Work out the finished part from the listing and answer in its coordinate system (mm). Face numbers are marked on the shaded views. A direction names the side the tool comes from. Coordinates: 2 decimals unless noted, no trailing zeros. Write each loop counter-clockwise with the first axis right and the second up, starting at its lowest first coordinate (ties: lowest second). Pieces come first, ordered by that corner, then holes. Notation, with made-up numbers: (-22.75, 8.5) - (12.25, 8.5) arc R18 cw to (12.25, 33.5) - close; hole circle Ø3 at (30, 51.5). An arc over 180 degrees is marked (long way). One line per item, written item: value.
```python
from build123d import *

# Parameters (mm, degrees)
ESQUISSE1_W             = 28
ESQUISSE1_H             = 23
BOSS_EXTRU_1_DEPTH      = 2
ESQUISSE2_R             = 2
ENL_V_MAT_EXTRU_1_DEPTH = 37.290494623
CHANFREIN1_SIZE         = 1


with BuildPart() as part:
    # Esquisse1 → Boss.-Extru.1 (new body)
    with BuildSketch(Plane.XY):
        with Locations((14, 11.5)):
            Rectangle(ESQUISSE1_W, ESQUISSE1_H)
    extrude(amount=BOSS_EXTRU_1_DEPTH)

    # Esquisse2 → Enlèv. mat.-Extru.1 (cut, through all)
    with BuildSketch(Plane.XY.offset(2)):
        with Locations((6, 4)):
            Circle(ESQUISSE2_R)
        with Locations(Location((22, 4, 0), (0, 0, 180))):
            Circle(ESQUISSE2_R)
        with BuildLine():
            Line((8.2, 19), (8.2, 15))
            ThreePointArc((8.2, 15), (6, 12.8), (3.8, 15))
            Line((3.8, 15), (3.8, 19))
            ThreePointArc((3.8, 19), (6, 21.2), (8.2, 19))
        make_face()
        with BuildLine():
            Line((19.8, 19), (19.8, 15))
            ThreePointArc((19.8, 15), (22, 12.8), (24.2, 15))
            Line((24.2, 15), (24.2, 19))
            ThreePointArc((24.2, 19), (22, 21.2), (19.8, 19))
        make_face()
    extrude(amount=-ENL_V_MAT_EXTRU_1_DEPTH, mode=Mode.SUBTRACT)

    # Chanfrein1
    chanfrein1_edges = [part.edges().sort_by_distance(p)[0] for p in [
        (0, 23, 1),
        (28, 23, 1),
        (28, 0, 1),
        (0, 0, 1),
    ]]
    chamfer(chanfrein1_edges, length=CHANFREIN1_SIZE)


solid = part.part
```
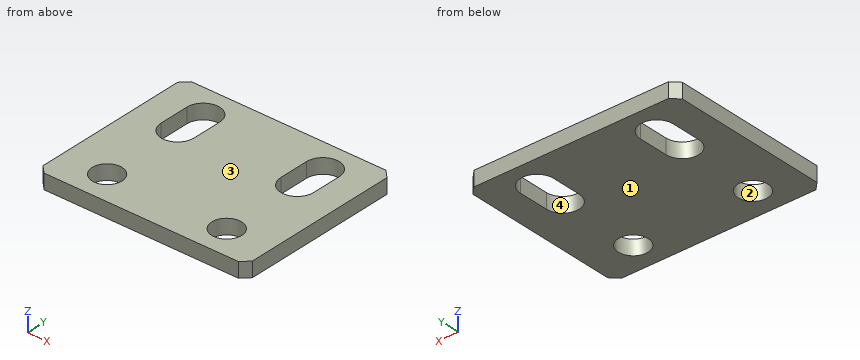
Item 1: Determine the mould class of the marked faces 1 and 2 for opening direction X: +X half, -X half, draft (parallel to the pull), parting line (faces both ways), or undercut.
Evaluation:
face 1: draft
face 2: undercut
Item 2: Section A-A, the plane x = 22 is taken. Determine the outline of the cut face in (y, z), then the cut area to 3 significant figures.
Evaluation:
outline: (0, 0) - (2, 0) - (2, 2) - (0, 2) - close; (6, 0) - (12.8, 0) - (12.8, 2) - (6, 2) - close; (21.2, 0) - (23, 0) - (23, 2) - (21.2, 2) - close
area: 21.2 mm2
Item 3: Consider probe 1 along X at (y, z) = (16, 0.65); probe 2 along Y at (x, z) = (22, 1.4); probe 3 along Y at (x, z) = (21.5, 0.9). Determine where each line is inside the solid, lowest interval first.
Evaluation:
probe 1: x = 0 to 3.8, 8.2 to 19.8, 24.2 to 28
probe 2: y = 0 to 2, 6 to 12.8, 21.2 to 23
probe 3: y = 0 to 2.06, 5.94 to 12.86, 21.14 to 23
Item 4: Section C-C, the plane z = 0.6 is taken. Determine the outline of the cut face in (x, y).
Evaluation:
outline: (0, 1) - (1, 0) - (27, 0) - (28, 1) - (28, 22) - (27, 23) - (1, 23) - (0, 22) - close; hole (3.8, 15) arc R2.2 ccw to (8.2, 15) - (8.2, 19) arc R2.2 ccw to (3.8, 19) - close; hole circle Ø4 at (6, 4); hole (19.8, 15) arc R2.2 ccw to (24.2, 15) - (24.2, 19) arc R2.2 ccw to (19.8, 19) - close; hole circle Ø4 at (22, 4)
Item 5: Section B-B, the plane y = 17.5 is taken. Determine the outline of the cut face in (x, z).
Evaluation:
outline: (0, 0) - (3.8, 0) - (3.8, 2) - (0, 2) - close; (8.2, 0) - (19.8, 0) - (19.8, 2) - (8.2, 2) - close; (24.2, 0) - (28, 0) - (28, 2) - (24.2, 2) - close
Item 6: Which of the six approach directions +Z, -Z, +X, -X, +Y, -Y give full straight-line access (tool end or side, diameter ignored) to the marked faces 3 and 4?
Evaluation:
face 3: +Z, +X, -X, +Y, -Y
face 4: +Z, -Z
